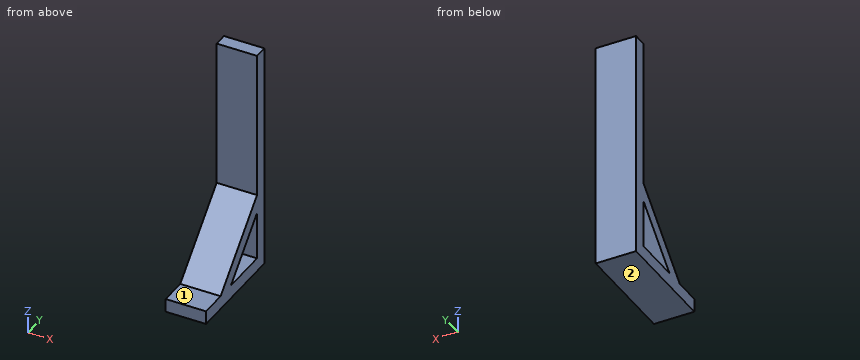
from build123d import *

# Parameters (mm, degrees)
BOSS_EXTRUDE1_DEPTH = 76.2


with BuildPart() as part:
    # Sketch1 → Boss-Extrude1 (new body)
    with BuildSketch(Plane(origin=(0, 0, 0), x_dir=(0, 0, -1), z_dir=(1, 0, 0))):
        Polygon((0, 0), (0, 203.2), (-431.8, 203.2), (-431.8, 177.8), (-152.4, 177.8), (-25.4, 50.8), (-25.4, 0), align=None)
        Polygon((-116.478975516, 177.8), (-25.4, 177.8), (-25.4, 86.721024484), align=None, mode=Mode.SUBTRACT)
    extrude(amount=BOSS_EXTRUDE1_DEPTH)


solid = part.part
Build history of the part. All positions in model axes, mm. Face numbers are marked on the shaded views. A direction names the side the tool comes from. Give positions to 0.01 mm unless a question says otherwise; leave off trailing zeros. Order: outer loops, then holes, each group sorted by start corner. A loop starts at its lowest first (then second) coordinate and runs counter-clockwise, first axis right, second up. Notation, with made-up numbers: M 57,83 L 69,83 A32 ccw 69,121 Z; hole C 89.25,44.25 d8. An arc over 180 degrees is marked long. Use one line per item in the form item = value.
1) Saw through at A-A (x = 35.5). Give the cut face in (y, z).
Calculated:
outline = M 0,0 L 203.2,0 L 203.2,431.8 L 177.8,431.8 L 177.8,152.4 L 50.8,25.4 L 0,25.4 Z; hole M 86.72,25.4 L 177.8,25.4 L 177.8,116.48 Z
2) Probe probe 1 along Y at (x, z) = (14.5, 187.5); probe 2 along Z at (x, y) = (58.5, 11); probe 3 along Z at (x, y) = (13.5, 164). List the from-to ranges inside material, lowest first.
Calculated:
probe_1 = 177.8 to 203.2
probe_2 = 0 to 25.4
probe_3 = 0 to 25.4, 102.68 to 138.6
3) Saw through at C-C (z = 32). Give the cut face in (x, y), plus the area to 3 significant figures.
Calculated:
outline = M 0,57.4 L 76.2,57.4 L 76.2,93.32 L 0,93.32 Z; M 0,177.8 L 76.2,177.8 L 76.2,203.2 L 0,203.2 Z
area = 4,670 mm2
4) Saw through at D-D (y = 17.5). Give the cut face in (x, z).
Calculated:
outline = M 0,0 L 76.2,0 L 76.2,25.4 L 0,25.4 Z
5) Saw through at B-B (y = 140.5). Give the cut face in (x, z).
Calculated:
outline = M 0,0 L 76.2,0 L 76.2,25.4 L 0,25.4 Z; M 0,79.18 L 76.2,79.18 L 76.2,115.1 L 0,115.1 Z
6) Drop flat-ended pins along their axis: pin 1 (5 mm diameter, centred on x = 25.5, z = 293.5, fed in from -Y); pin 2 (15 mm diameter, centred on x = 20, y = 33, fed in from +Z); pin 3 (5 mm diameter, centred on x = 66.5, z = 76, fed in from -Y). Give the stop position or say it passes through.
Calculated:
pin_1 = 177.8
pin_2 = 25.4
pin_3 = 98.9
7) Tool access for the marked faces 1 and 2: list every direction of +Z, -Z, +X, -X, +Y, -Y with a clear straight run to the whole face (end or side of a thin tool).
Calculated:
face_1 = +Z, +X, -X, -Y
face_2 = -Z, +X, -X, +Y, -Y
